Could you check a few things on this model? Use its own coordinates, in mm. A direction names the side the tool comes from. Give positions to 0.01 mm unless a question says otherwise; leave off trailing zeros. Order: outer loops, then holes, each group sorted by start corner. A loop starts at its lowest first (then second) coordinate and runs counter-clockwise, first axis right, second up.
(1) Imagine slicing it at D-D, the plane x = 4.5. Write out the boundary of the cut face in (y, z).
(2) Imagine slicing it at B-B, the plane z = 16.5. State how many separate pieces and enclosed holes the cut face has, then the cut area to 3 significant figures.
(3) On a 3-axis mill with a long thin cutter (end or side, diameter ignored), from which of +Z, -Z, +X, -X, +Y, -Y can I reach the whole of each face in a straight line? I mean faces 5 (the flat face through (3, -35.9, 12)), 6 (the flat face through (0, -37.5, 12)), 7 (the cylindrical face through (0.672, -28.446, 11.154)). Say none if no direction works.
(4) If I drill on probe 1 along X at (y, z) = (10, 12); probe 2 along Y at (x, z) = (0, 8.75); probe 3 along X at (y, z) = (28.5, 17.5), over which ranges is the centre line in solid material (lowest first)?
(5) Imagine slicing it at A-A, the plane y = -29.5. Write out the boundary of the cut face in (x, z).
(6) Will these pins go through, and if not, where does the flat tip stop? pin 1 (3 mm diameter, centred on y = 34, z = 8, fed in from -X); pin 2 (4 mm diameter, centred on x = -3.5, z = 11.5, fed in from +Y); pin 3 (8 mm diameter, centred on y = -2, z = 18.5, fed in from +X).
(7) Imagine slicing it at C-C, the plane y = 21. Write out the boundary of the cut face in (x, z).
(8) If we mould it in two halves opening along Y, with no side actions, what happens to faces 1 (the flat face through (0.8, -34, 12)), 2 (the cylindrical face through (-15.1, -49.14, 1.13)), 3 (the flat face through (-7.35, -1, 12)), 4 (the flat face through (-3, 0.8, 12))? For each: released by +Y, released by -Y, zero draft, split by the parting line, or undercut.
from build123d import *

# Parameters (mm, degrees)
EXTRUDE_2_DEPTH     = 22
EXTRUDE_3_DEPTH     = 2.3
SHELL_1_T           = -1.6
EXTRUDE_4_DEPTH     = 20.4
EXTRUDE_START       = -20.4
SKETCH_4_R          = 2.75
SKETCH_4_R_2        = 1.25
EXTRUDE_5_DEPTH     = 20.4
SKETCH_5_R          = 1.25
CUT_EXTRUDE_1_DEPTH = 22
SKETCH_6_R          = 0.5
EXTRUDE_6_DEPTH     = 1.3


with BuildPart() as part:
    # 스케치1 → 보스-돌출2 (new body)
    with BuildSketch(Plane(origin=(0, 0, 0), x_dir=(0, 1, 0), z_dir=(0, 0, 1))):
        with BuildLine():
            Line((-36.5, 7.35), (36.5, 7.35))
            ThreePointArc((36.5, 7.35), (37.207106781, 7.057106781), (37.5, 6.35))
            Line((37.5, 6.35), (37.5, -6.35))
            ThreePointArc((37.5, -6.35), (37.207106781, -7.057106781), (36.5, -7.35))
            Line((36.5, -7.35), (-36.5, -7.35))
            ThreePointArc((-36.5, -7.35), (-37.207106781, -7.057106781), (-37.5, -6.35))
            Line((-37.5, -6.35), (-37.5, 6.35))
            ThreePointArc((-37.5, 6.35), (-37.207106781, 7.057106781), (-36.5, 7.35))
        make_face()
    extrude(amount=EXTRUDE_2_DEPTH)

    # 스케치1<5> → 보스-돌출3 (add)
    with BuildSketch(Plane(origin=(0, 0, 0), x_dir=(0, 1, 0), z_dir=(0, 0, 1))):
        with BuildLine():
            Line((-47, 16), (47, 16))
            ThreePointArc((47, 16), (49.121320344, 15.121320344), (50, 13))
            Line((50, 13), (50, -13))
            ThreePointArc((50, -13), (49.121320344, -15.121320344), (47, -16))
            Line((47, -16), (-47, -16))
            ThreePointArc((-47, -16), (-49.121320344, -15.121320344), (-50, -13))
            Line((-50, -13), (-50, 13))
            ThreePointArc((-50, 13), (-49.121320344, 15.121320344), (-47, 16))
        make_face()
        with BuildLine():
            Line((-36.5, 7.35), (36.5, 7.35))
            ThreePointArc((36.5, 7.35), (37.207106781, 7.057106781), (37.5, 6.35))
            Line((37.5, 6.35), (37.5, -6.35))
            ThreePointArc((37.5, -6.35), (37.207106781, -7.057106781), (36.5, -7.35))
            Line((36.5, -7.35), (-36.5, -7.35))
            ThreePointArc((-36.5, -7.35), (-37.207106781, -7.057106781), (-37.5, -6.35))
            Line((-37.5, -6.35), (-37.5, 6.35))
            ThreePointArc((-37.5, 6.35), (-37.207106781, 7.057106781), (-36.5, 7.35))
        make_face(mode=Mode.SUBTRACT)
    extrude(amount=EXTRUDE_3_DEPTH)

    # 쉘1
    shell_1_openings = [part.faces().sort_by_distance(p)[0] for p in [
        (0, 0, 22),
    ]]
    offset(amount=SHELL_1_T, openings=shell_1_openings, kind=Kind.INTERSECTION)

    # 스케치3 → 보스-돌출4 (add)
    with BuildSketch(Plane.XY.offset(1.6)):
        Polygon((0.8, 35.9), (0.8, 0.8), (5.75, 0.8), (5.75, -0.8), (0.8, -0.8), (0.8, -35.9), (-0.8, -35.9), (-0.8, -0.8), (-5.75, -0.8), (-5.75, 0.8), (-0.8, 0.8), (-0.8, 35.9), align=None)
    extrude(amount=EXTRUDE_4_DEPTH)

    # 스케치4 → 보스-돌출5 (add)
    with BuildSketch(Plane.XY.offset(22).offset(EXTRUDE_START)):
        with Locations((0, 29.5)):
            Circle(SKETCH_4_R)
        with Locations((0, 29.5)):
            Circle(SKETCH_4_R_2, mode=Mode.SUBTRACT)
        with Locations((0, -29.5)):
            Circle(SKETCH_4_R)
    extrude(amount=EXTRUDE_5_DEPTH)

    # 스케치5 → 컷-돌출1 (cut)
    with BuildSketch(Plane.XY.offset(22)):
        with Locations((0, -29.5)):
            Circle(SKETCH_5_R)
        with Locations((0, 29.5)):
            Circle(SKETCH_5_R)
    extrude(amount=-CUT_EXTRUDE_1_DEPTH, mode=Mode.SUBTRACT)

    # 스케치6 → 보스-돌출6 (add)
    with BuildSketch(Plane.XY.offset(22)):
        with Locations((-6.55, -32.2)):
            Circle(SKETCH_6_R)
        with Locations((6.55, -15.5)):
            Circle(SKETCH_6_R)
        with Locations((-6.55, 32.2)):
            Circle(SKETCH_6_R)
        with Locations((6.55, 15.5)):
            Circle(SKETCH_6_R)
    extrude(amount=EXTRUDE_6_DEPTH)


solid = part.part
Answer block:
1. outline: (-50, 0) - (50, 0) - (50, 2.3) - (37.5, 2.3) - (37.5, 22) - (35.9, 22) - (35.9, 1.6) - (0.8, 1.6) - (0.8, 22) - (-0.8, 22) - (-0.8, 1.6) - (-35.9, 1.6) - (-35.9, 22) - (-37.5, 22) - (-37.5, 2.3) - (-50, 2.3) - close
2. separate pieces: 1
2. enclosed holes: 6
2. area: 427 mm2
3. face 5: +Z
3. face 6: +Z, +X, -X, -Y
3. face 7: +Z, -Z
4. probe 1: x = -7.35 to -5.75, -0.8 to 0.8, 5.75 to 7.35
4. probe 2: y = -37.5 to -30.75, -28.25 to 28.25, 30.75 to 37.5
4. probe 3: x = -7.35 to -5.75, -2.56 to -0.75, 0.75 to 2.56, 5.75 to 7.35
5. outline: (-16, 0) - (-1.25, 0) - (-1.25, 22) - (-2.75, 22) - (-2.75, 1.6) - (-5.75, 1.6) - (-5.75, 22) - (-7.35, 22) - (-7.35, 2.3) - (-16, 2.3) - close; (1.25, 0) - (16, 0) - (16, 2.3) - (7.35, 2.3) - (7.35, 22) - (5.75, 22) - (5.75, 1.6) - (2.75, 1.6) - (2.75, 22) - (1.25, 22) - close
6. pin 1: stops at x = -7.35
6. pin 2: stops at y = 37.5
6. pin 3: stops at x = 7.35
7. outline: (-16, 0) - (16, 0) - (16, 2.3) - (7.35, 2.3) - (7.35, 22) - (5.75, 22) - (5.75, 1.6) - (0.8, 1.6) - (0.8, 22) - (-0.8, 22) - (-0.8, 1.6) - (-5.75, 1.6) - (-5.75, 22) - (-7.35, 22) - (-7.35, 2.3) - (-16, 2.3) - close
8. face 1: undercut
8. face 2: released by -Y
8. face 3: zero draft
8. face 4: undercut
